```python
from build123d import *

# Parameters (mm, degrees)
SKETCH1_W           = 50
SKETCH1_H           = 54.105
BOSS_EXTRUDE1_DEPTH = 12
SKETCH2_R           = 3.15
CUT_EXTRUDE1_DEPTH  = 75.641483272
FILLET1_R           = 8
SKETCH3_R           = 11
SKETCH3_R_2         = 1.7
CUT_EXTRUDE2_DEPTH  = 75.641483272
CUT_EXTRUDE4_DEPTH  = 8


with BuildPart() as part:
    # Sketch1 → Boss-Extrude1 (new body)
    with BuildSketch(Plane.XY):
        with Locations((25, 27.0525)):
            Rectangle(SKETCH1_W, SKETCH1_H)
    extrude(amount=BOSS_EXTRUDE1_DEPTH)

    # Sketch2 → Cut-Extrude1 (cut, through all)
    with BuildSketch(Plane(origin=(0, 0, 0), x_dir=(0, 0, -1), z_dir=(1, 0, 0))):
        with Locations((-6, 46.105)):
            Circle(SKETCH2_R)
        with Locations(Location((-6, 8, 0), (0, 0, 180))):
            Circle(SKETCH2_R)
    extrude(amount=CUT_EXTRUDE1_DEPTH, mode=Mode.SUBTRACT)

    # Fillet1
    fillet1_edges = [part.edges().sort_by_distance(p)[0] for p in [
        (25, 54.105, 0),
        (25, 0, 0),
    ]]
    fillet(fillet1_edges, radius=FILLET1_R)

    # Sketch3 → Cut-Extrude2 (cut, through all)
    with BuildSketch(Plane(origin=(0, 0, 0), x_dir=(-1, 0, 0), z_dir=(0, 0, -1))):
        with Locations((-32, 27.0525)):
            Circle(SKETCH3_R)
        with Locations((-19, 40.0525)):
            Circle(SKETCH3_R_2)
        with Locations((-19, 14.0525)):
            Circle(SKETCH3_R_2)
        with Locations((-45, 14.0525)):
            Circle(SKETCH3_R_2)
        with Locations((-45, 40.0525)):
            Circle(SKETCH3_R_2)
        with BuildLine():
            Line((-8.5, 0), (-8.5, 24.282572203))
            ThreePointArc((-8.5, 24.282572203), (-10.15, 27.0525), (-8.5, 29.822427797))
            Line((-8.5, 29.822427797), (-8.5, 33.0525))
            ThreePointArc((-8.5, 33.0525), (-7, 34.5525), (-5.5, 33.0525))
            Line((-5.5, 33.0525), (-5.5, 29.822427797))
            ThreePointArc((-5.5, 29.822427797), (-3.85, 27.0525), (-5.5, 24.282572203))
            Line((-5.5, 24.282572203), (-5.5, 0))
            Line((-5.5, 0), (-8.5, 0))
        make_face()
    extrude(amount=-CUT_EXTRUDE2_DEPTH, mode=Mode.SUBTRACT)

    # Sketch5 → Cut-Extrude4 (cut)
    with BuildSketch(Plane(origin=(0, 0, 0), x_dir=(-1, 0, 0), z_dir=(0, 0, -1))):
        with BuildLine():
            Line((-19, 17.6525), (-14, 17.6525))
            Line((-14, 17.6525), (-14, 36.4525))
            Line((-14, 36.4525), (-19, 36.4525))
            ThreePointArc((-19, 36.4525), (-21.510876341, 37.472674425), (-22.598679445, 39.955))
            Line((-22.598679445, 39.955), (-22.598679445, 41.7525))
            Line((-22.598679445, 41.7525), (-41.401320555, 41.7525))
            Line((-41.401320555, 41.7525), (-41.401320555, 39.955))
            ThreePointArc((-41.401320555, 39.955), (-42.489123659, 37.472674425), (-45, 36.4525))
            Line((-45, 36.4525), (-50, 36.4525))
            Line((-50, 36.4525), (-50, 17.6525))
            Line((-50, 17.6525), (-45, 17.6525))
            ThreePointArc((-45, 17.6525), (-42.489123659, 16.632325575), (-41.401320555, 14.15))
            Line((-41.401320555, 14.15), (-41.401320555, 12.3525))
            Line((-41.401320555, 12.3525), (-22.598679445, 12.3525))
            Line((-22.598679445, 12.3525), (-22.598679445, 14.15))
            ThreePointArc((-22.598679445, 14.15), (-21.510876341, 16.632325575), (-19, 17.6525))
        make_face()
    extrude(amount=-CUT_EXTRUDE4_DEPTH, mode=Mode.SUBTRACT)


solid = part.part
```
Source: CAD feature listing. Evaluate the final solid. Frame: model axes, mm. A direction names the side the tool comes from. Coordinates: 2 decimals unless noted, no trailing zeros. Write each loop counter-clockwise with the first axis right and the second up, starting at its lowest first coordinate (ties: lowest second). Pieces come first, ordered by that corner, then holes. Notation, with made-up numbers: (-37, 48) -> (12, 48) arc R15 ccw to (12, 65) -> close; hole circle Ø1 at (44, 9.25). An arc over 180 degrees is marked (long way). Return JSON: item names as keys, results as strings. Group by question number.
1) Set-up query: faces 5 (the face through (22.599, 41, 4)), 6 (the face through (8.5, 31, 6)), 7 (the face through (21.51, 30.36, 9.97)), 8 (the face through (47, 36.452, 4)). Return all of +Z, -Z, +X, -X, +Y, -Y with unobstructed straight access to the full face (end or side cutting, diameter ignored); none if empty.
2) Ray query, line 1 along X through (y, z) = (27, 2.5); line 2 along X through (y, z) = (38.5, 11); line 3 along X through (y, z) = (3, 4.5). Return the intervals inside material, ascending.
3) Section query A-A, the plane x = 32. State how many separate pieces and enclosed holes the cut face has, plus the area to 3 significant figures.
4) Mould query, pull axis X, two halves, no side actions, for faces 1 (the face through (0, 27, 6)), 2 (the face through (17, 17.652, 4)), 3 (the face through (41.401, 13, 4)), 4 (the face through (17.43, 13.4, 5.92)). Classes: +X half, -X half, draft (parallel to the pull), parting line (faces both ways), or undercut.
5) Section query C-C, the plane y = 31.5. Return loops of the section in (x, z).
6) Contact query for flat-ended pins moving along their axis: P1, Ø3, axis at x = 45, y = 40.05, coming from the -Z side; P2, Ø2.5, axis at x = 17, z = 4, coming from the +Y side; P3, Ø1.5, axis at x = 17, z = 6, coming from the -Y side. Output: stop coordinate, or through.
From the geometry:
{
 "1": {"face 5": "-Z", "face 6": "+Z, -Z, -Y", "face 7": "+Z, -Z", "face 8": "-Z, +X"},
 "2": {"line 1": "0 to 3.85, 10.15 to 14", "line 2": "0 to 18.31, 19.69 to 44.31, 45.69 to 50", "line 3": "0 to 5.5, 8.5 to 50"},
 "3": {"separate pieces": "2", "enclosed holes": "2", "area": "236 mm²"},
 "4": {"face 1": "-X half", "face 2": "draft", "face 3": "undercut", "face 4": "undercut"},
 "5": {"outline": "(0, 0) -> (5.5, 0) -> (5.5, 12) -> (0, 12) -> close; (8.5, 0) -> (14, 0) -> (14, 8) -> (21.94, 8) -> (21.94, 12) -> (8.5, 12) -> close; (42.06, 8) -> (50, 8) -> (50, 12) -> (42.06, 12) -> close"},
 "6": {"P1": "through", "P2": "y = 53.62", "P3": "y = 0.1"}
}
